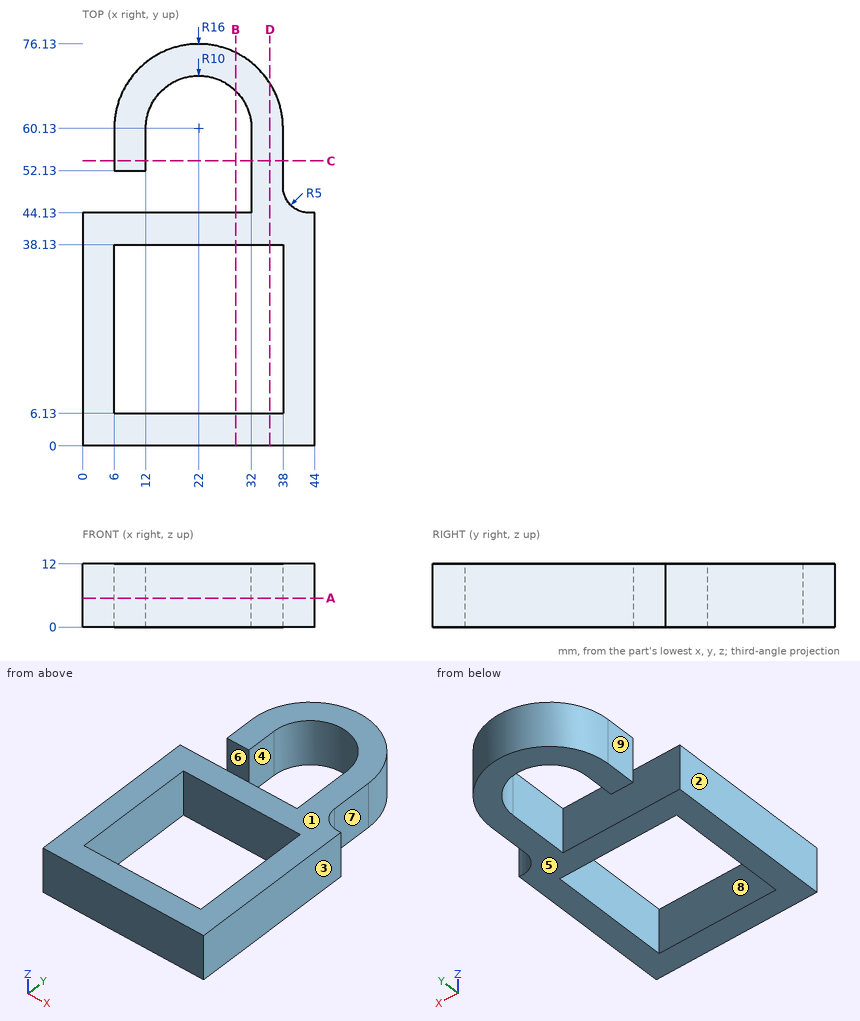
Job drawing, mm, ordinate dimensions from the low corner. One solid piece. A direction names the side the tool comes from. Give positions to 0.01 mm unless a question says otherwise; leave off trailing zeros. Loops run counter-clockwise (first coordinate to the right, second up) from the corner with the lowest first, then second, coordinate; pieces in that order, holes last. Notation, with made-up numbers: (21.5, 0.5) -> (55.5, 0.5) arc R18 cw to (55.5, 34.5) -> close; hole circle Ø6 at (-30.75, 15). An arc over 180 degrees is marked (long way). Use a Markdown table: item, result. Add a question column.
(1) Wall check: line 1 along X through (y, z) = (17.5, 6); line 2 along Y through (x, z) = (21, 2.75); line 3 along Y through (x, z) = (28, 4.5). Give the ranges that are in metal, low to high.
(2) Slice it at A-A on z = 5.5. List the corners of the cut face in (x, y), and give its area (3 significant figures).
(3) Slice it at C-C on y = 54. List the corners of the cut face in (x, z), and give its area (3 significant figures).
(4) Tool access for the marked faces 5, 6, 7, 8 and 9: list every direction of +Z, -Z, +X, -X, +Y, -Y with a clear straight run to the whole face (end or side of a thin tool).
(5) Mould opens along X. For the marked faces 1, 2, 3 and 4 say: +X half, -X half, draft (parallel to the pull), parting line (faces both ways), or undercut.
(6) Drop flat-ended pins along their axis: pin 1 Ø0.8 at (x, z) = (43.5, 4) entering from +Y; pin 2 Ø1.5 at (x, z) = (28.5, 2.5) entering from +Y; pin 3 Ø6.5 at (x, z) = (9, 5) entering from -Y; pin 4 Ø6 at (y, z) = (59.5, 7.5) entering from +X. Give the stop position or say it passes through.
(7) Slice it at D-D on x = 35.5. List the corners of the cut face in (y, z), and give its area (3 significant figures).
(8) Slice it at B-B on x = 29. List the corners of the cut face in (y, z).
Filled sheet:
| question | item | result |
|---|---|---|
| 1 | line 1 | 0 to 6, 38 to 44 |
| 1 | line 2 | 0 to 6.13, 38.13 to 44.13, 70.08 to 76.1 |
| 1 | line 3 | 0 to 6.13, 38.13 to 44.13, 68.13 to 74.96 |
| 2 | outline | (0, 0) -> (44, 0) -> (44, 44.13) -> (43, 44.13) arc R5 cw to (38, 49.13) -> (38, 60.13) arc R16 ccw to (6, 60.13) -> (6, 52.13) -> (12, 52.13) -> (12, 60.13) arc R10 cw to (32, 60.13) -> (32, 44.13) -> (0, 44.13) -> close; hole (6, 6.13) -> (38, 6.13) -> (38, 38.13) -> (6, 38.13) -> close |
| 2 | area | 1,310 mm2 |
| 3 | outline | (6, 0) -> (12, 0) -> (12, 12) -> (6, 12) -> close; (32, 0) -> (38, 0) -> (38, 12) -> (32, 12) -> close |
| 3 | area | 144 mm2 |
| 4 | face 5 | -Z, +X, -X, +Y, -Y |
| 4 | face 6 | +Z, -Z, -X |
| 4 | face 7 | +Z, -Z, +X, +Y |
| 4 | face 8 | +Z, -Z |
| 4 | face 9 | +Z, -Z, -X, +Y |
| 5 | face 1 | draft |
| 5 | face 2 | -X half |
| 5 | face 3 | +X half |
| 5 | face 4 | undercut |
| 6 | pin 1 | y = 44.13 |
| 6 | pin 2 | y = 75.06 |
| 6 | pin 3 | y = 0 |
| 6 | pin 4 | x = 38 |
| 7 | outline | (0, 0) -> (6.13, 0) -> (6.13, 12) -> (0, 12) -> close; (38.13, 0) -> (68.72, 0) -> (68.72, 12) -> (38.13, 12) -> close |
| 7 | area | 441 mm2 |
| 8 | outline | (0, 0) -> (6.13, 0) -> (6.13, 12) -> (0, 12) -> close; (38.13, 0) -> (44.13, 0) -> (44.13, 12) -> (38.13, 12) -> close; (67.27, 0) -> (74.52, 0) -> (74.52, 12) -> (67.27, 12) -> close |
